The model under review builds one solid part; all positions refer to its coordinate system, in mm. A direction names the side the tool comes from. Coordinates: 2 decimals unless noted, no trailing zeros. Loops run counter-clockwise (first coordinate to the right, second up) from the corner with the lowest first, then second, coordinate; pieces in that order, holes last. Notation, with made-up numbers: M 6,-29.75 L 22,-29.75 A17 ccw 22,-3.75 Z; hole C -20.75,27.25 d6. An arc over 180 degrees is marked long. Use one line per item in the form item = value.
```python
from build123d import *

# Parameters (mm, degrees)
SKETCH1_W           = 5.842
SKETCH1_H           = 5.842
BOSS_EXTRUDE1_DEPTH = 3.175


with BuildPart() as part:
    # Sketch1 → Boss-Extrude1 (new body)
    with BuildSketch(Plane(origin=(0, 0, 0), x_dir=(1, 0, 0), z_dir=(0, 1, 0))):
        Polygon((9.779, 38.1), (0, 38.1), (0, 0), (9.779, 0), (9.779, 9.271), (15.621, 9.271), (15.621, 0), (25.4, 0), (25.4, 38.1), (15.621, 38.1), (15.621, 28.575), (9.779, 28.575), align=None)
        with Locations((12.7, 19.05)):
            Rectangle(SKETCH1_W, SKETCH1_H, mode=Mode.SUBTRACT)
    extrude(amount=BOSS_EXTRUDE1_DEPTH)


solid = part.part
```
1. The part is to be moulded in two halves that separate along X. For faces 1 (the face through (20, 2, 0)), 2 (the face through (0, 2, -19)), 3 (the face through (15.621, 2, -19)), 4 (the face through (9.779, 2, -5)), say which applies: pulls with the +X half, pulls with the -X half, needs draft (parallel to the pull), parting line crosses it, or undercut.
Response values:
face_1 = needs draft
face_2 = pulls with the -X half
face_3 = undercut
face_4 = undercut
2. Insertion check: P1, Ø1.6, axis at x = 12, y = 1, coming from the +Z side; P2, Ø1, axis at x = 13, y = 2, coming from the -Z side (3 decimals). Each pin has a flat end and moves straight along its axis. Give the tip position at first contact, or say it passes through.
Response values:
P1 = -9.27
P2 = -28.575
3. Add section B-B (z = -33.5). State the section outline as (x, y) points (3 decimals), then the cut area to 3 significant figures.
Response values:
outline = M 0,0 L 9.779,0 L 9.779,3.175 L 0,3.175 Z; M 15.621,0 L 25.4,0 L 25.4,3.175 L 15.621,3.175 Z
area = 62.1 mm^2
4. Add section C-C (y = 0.7). State the section outline as (x, z) points (3 decimals).
Response values:
outline = M 0,-38.1 L 9.779,-38.1 L 9.779,-28.575 L 15.621,-28.575 L 15.621,-38.1 L 25.4,-38.1 L 25.4,0 L 15.621,0 L 15.621,-9.271 L 9.779,-9.271 L 9.779,0 L 0,0 Z; hole M 9.779,-21.971 L 15.621,-21.971 L 15.621,-16.129 L 9.779,-16.129 Z
5. Machinability: for faces 5 (the face through (13, 2, -21.971)), 6 (the face through (13, 2, -28.575)), 7 (the face through (13, 2, -9.271)), which of the approach directions +Z, -Z, +X, -X, +Y, -Y give a long, thin tool a straight path to every point of the face, cutting with its end or side? Answer none if there is none.
Response values:
face_5 = +Y, -Y
face_6 = -Z, +Y, -Y
face_7 = +Z, +Y, -Y
6. Add section A-A (x = 12.25). State the section outline as (y, z) points (3 decimals).
Response values:
outline = M 0,-28.575 L 3.175,-28.575 L 3.175,-21.971 L 0,-21.971 Z; M 0,-16.129 L 3.175,-16.129 L 3.175,-9.271 L 0,-9.271 Z
7. Wall thickness on line 1 along X through (y, z) = (1.7, -19.5); line 2 along Z through (x, y) = (15.5, 2.75) (3 decimals): over which ranges is each line inside the solid? List them lowest first. Write a range as from..to.
Response values:
line_1 = 0..9.78, 15.62..25.4
line_2 = -28.575..-21.971, -16.129..-9.271
